```python
from build123d import *


with BuildPart() as part:
    # Esquisse1 → Révolution1 (revolve)
    with BuildSketch(Plane.XY):
        with BuildLine():
            Line((-3.25, -1.4), (-3.25, -2))
            ThreePointArc((-3.25, -2), (-3.103553391, -2.353553391), (-2.75, -2.5))
            Line((-2.75, -2.5), (-1.48, -2.5))
            Line((-1.48, -2.5), (-1.48, 2.5))
            Line((-1.48, 2.5), (-2.75, 2.5))
            ThreePointArc((-2.75, 2.5), (-3.103553391, 2.353553391), (-3.25, 2))
            Line((-3.25, 2), (-3.25, 1.4))
            Line((-3.25, 1.4), (-2.13, 1.4))
            Line((-2.13, 1.4), (-2.13, -1.4))
            Line((-2.13, -1.4), (-3.25, -1.4))
        make_face()
    revolve(axis=Axis((0, 0, 0), (0, 1, 0)))


solid = part.part
```
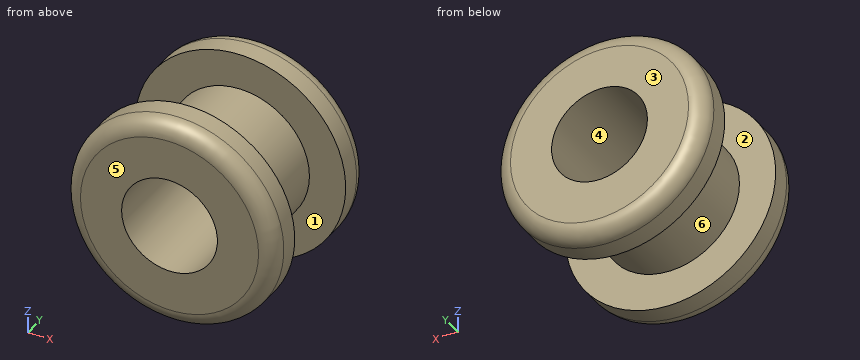
Build history of the part. All positions in model axes, mm. Face numbers are marked on the shaded views. A direction names the side the tool comes from. Give positions to 0.01 mm unless a question says otherwise; leave off trailing zeros. Loops run counter-clockwise (first coordinate to the right, second up) from the corner with the lowest first, then second, coordinate; pieces in that order, holes last.
1) Band-saw the part on A-A on x = 0. List the corners of the cut face in (y, z).
Values follow:
outline: (-2.5, -2.75) arc R0.5 ccw to (-2, -3.25) - (-1.4, -3.25) - (-1.4, -2.13) - (1.4, -2.13) - (1.4, -3.25) - (2, -3.25) arc R0.5 ccw to (2.5, -2.75) - (2.5, -1.48) - (-2.5, -1.48) - close; (-2.5, 1.48) - (2.5, 1.48) - (2.5, 2.75) arc R0.5 ccw to (2, 3.25) - (1.4, 3.25) - (1.4, 2.13) - (-1.4, 2.13) - (-1.4, 3.25) - (-2, 3.25) arc R0.5 ccw to (-2.5, 2.75) - close
2) Band-saw the part on B-B on z = 0. List the corners of the cut face in (x, y).
Values follow:
outline: (-3.25, -2) arc R0.5 ccw to (-2.75, -2.5) - (-1.48, -2.5) - (-1.48, 2.5) - (-2.75, 2.5) arc R0.5 ccw to (-3.25, 2) - (-3.25, 1.4) - (-2.13, 1.4) - (-2.13, -1.4) - (-3.25, -1.4) - close; (1.48, -2.5) - (2.75, -2.5) arc R0.5 ccw to (3.25, -2) - (3.25, -1.4) - (2.13, -1.4) - (2.13, 1.4) - (3.25, 1.4) - (3.25, 2) arc R0.5 ccw to (2.75, 2.5) - (1.48, 2.5) - close
3) Probe line 1 along Z through (x, y) = (0, 1.2); line 2 along Z through (x, y) = (-1, -1.7); line 3 along Y through (x, z) = (0.5, -2.5). List the from-to ranges inside material, lowest first.
Values follow:
line 1: z = -2.13 to -1.48, 1.48 to 2.13
line 2: z = -3.09 to -1.09, 1.09 to 3.09
line 3: y = -2.5 to -1.4, 1.4 to 2.5
4) Band-saw the part on C-C on y = -0.6. List the corners of the cut face in (x, z), then the cut area to 3 significant figures.
Values follow:
outline: circle Ø4.26 at (0, 0); hole circle Ø2.96 at (0, 0)
area: 7.37 mm2
5) Two-plate mould, pull along Y, no slides. Class the marked faces 1, 2, 3 and 4: released by +Y, released by -Y, zero draft, split by the parting line, or undercut.
Values follow:
face 1: undercut
face 2: undercut
face 3: released by +Y
face 4: zero draft
6) Band-saw the part on D-D on y = 2.1. List the corners of the cut face in (x, z), then the cut area to 3 significant figures.
Values follow:
outline: circle Ø6.48 at (0, 0); hole circle Ø2.96 at (0, 0)
area: 26.1 mm2
7) 3-axis set-ups, long thin cutter, end or side, ignore diameter. For the marked faces 5 and 6: which of +Z, -Z, +X, -X, +Y, -Y reach the whole face in a straight line?
Values follow:
face 5: +Z, -Z, +X, -X, -Y
face 6: none
8) Drop flat-ended pins along their axis: P1, Ø3, axis at y = -0.5, z = 2, coming from the +X side; P2, Ø2, axis at x = 2, y = -1.5, coming from the +Z side; P3, Ø2.5, axis at x = 0, z = 0, coming from the +Y side. Give the stop position or say it passes through.
Values follow:
P1: stops at x = 3.15
P2: stops at z = 3.09
P3: passes through
